from build123d import *

# Parameters (mm, degrees)
SKETCH_1_W      = 110.5
SKETCH_1_H      = 66
EXTRUDE_1_DEPTH = 19
EXTRUDE_2_DEPTH = 19


with BuildPart() as part:
    # 草图1 → 凸台-拉伸1 (new body)
    with BuildSketch(Plane(origin=(0, 0, 0), x_dir=(1, 0, 0), z_dir=(0, 1, 0))):
        with Locations((55.25, -33)):
            Rectangle(SKETCH_1_W, SKETCH_1_H)
    extrude(amount=EXTRUDE_1_DEPTH)

    # 草图2 → 凸台-拉伸2 (add)
    with BuildSketch(Plane(origin=(0, 19, 0), x_dir=(1, 0, 0), z_dir=(0, 1, 0))):
        Polygon((110.5, 0), (45.531109974, 0), (59.21801075, 3.5), (110.5, 3.5), align=None)
    extrude(amount=-EXTRUDE_2_DEPTH)


solid = part.part
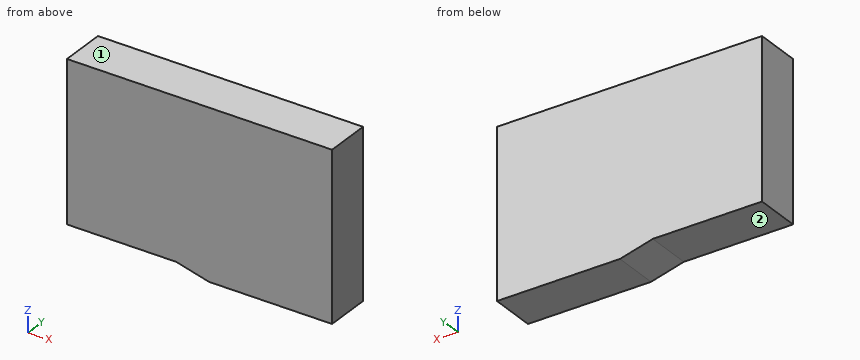
Work out the finished part from the listing and answer in its coordinate system (mm). Face numbers are marked on the shaded views. A direction names the side the tool comes from. Coordinates: 2 decimals unless noted, no trailing zeros. Loops run counter-clockwise (first coordinate to the right, second up) from the corner with the lowest first, then second, coordinate; pieces in that order, holes last. Notation, with made-up numbers: (-15, 56) -> (43, 56) arc R21 cw to (43, 79) -> close; hole circle Ø8 at (52, -3). An arc over 180 degrees is marked (long way). Answer as CSV lines item,"result".
1) The part is cut by section B-B (x = 39). Give the vertices of the cut face in (y, z).
A:
outline,"(0, 0) -> (19, 0) -> (19, 66) -> (0, 66) -> close"
2) The part is cut by section A-A (y = 10). Give the vertices of the cut face in (x, z).
A:
outline,"(0, 0) -> (45.53, 0) -> (59.22, -3.5) -> (110.5, -3.5) -> (110.5, 66) -> (0, 66) -> close"
3) Straight lines are drawn through the part: probe 1 along Z at (x, y) = (11, 13); probe 2 along Z at (x, y) = (50.5, 3.5). For each, find the intervals that lie inside material, in ascending order.
A:
probe 1,"z = 0 to 66"
probe 2,"z = -1.27 to 66"
4) For the marked faces 1 and 2, determine the directions among +Z, -Z, +X, -X, +Y, -Y from which every point of the face is accessible in a straight line to the end or side of a thin tool.
A:
face 1,"+Z, +X, -X, +Y, -Y"
face 2,"-Z, -X, +Y, -Y"
5) A flat-ended cylindrical pin translates along its axis: pin 1 (8 mm diameter, centred on x = 27, y = 8.5, fed in from -Z). Find the tip coordinate at first contact, or state that the pin passes through.
A:
pin 1,"stops at z = 0"
